Source: CAD feature listing. Evaluate the final solid. Frame: model axes, mm. A direction names the side the tool comes from. Round coordinates to 2 decimals unless told otherwise and drop trailing zeros. Loops run counter-clockwise (first coordinate to the right, second up) from the corner with the lowest first, then second, coordinate; pieces in that order, holes last. Notation, with made-up numbers: (-14, 8.25) -> (25, 8.25) arc R13 ccw to (25, 25.25) -> close; hole circle Ø4 at (46, 35). An arc over 180 degrees is marked (long way). Put each result on its own line as item: value. Start each with the question number.
1. Contact query for flat-ended pins moving along their axis: pin 1 (6 mm diameter, centred on y = 8.5, z = -19.5, fed in from +X); pin 2 (8 mm diameter, centred on y = 22.5, z = 22, fed in from -X); pin 3 (7 mm diameter, centred on x = -59, z = 2, fed in from +Y); pin 4 (3 mm diameter, centred on x = -58.17, z = 35.25, fed in from +Y). Output: stop coordinate, or through.
2. Set-up query: faces 1 (the flat face through (-56.101, 1.689, 47.074)), 2 (the flat face through (-64, 3, -1)). Return all of +Z, -Z, +X, -X, +Y, -Y with unobstructed straight access to the full face (end or side cutting, diameter ignored); none if empty.
3. Cut plane A-A (z = 0). Return the cut outline in (x, y), then the cut area to 3 significant figures.
4. Cut plane B-B (y = 31.5). Return the cut outline in (x, z).
5. Draft query along X for faces 3 (the conical face through (-85.33, 17.02, 0.83)), 4 (the cylindrical face through (-61.913, 1.479, 0.54)), 5 (the cylindrical face through (-59.74, 1.48, 35.9)), 6 (the cylindrical face through (-88.35, 35.92, -0.07)). Return one class per face: pulls with the +X half, pulls with the -X half, needs draft (parallel to the pull), parting line crosses it, or undercut.
6. Material intervals for L1, parallel to Y at x = -65.5, z = -9.5; L2, parallel to Z at x = -70, y = 5; L3, parallel to Y at x = -73.5, z = -21, sorted ascending.
```python
from build123d import *

# Parameters (mm, degrees)
R_VOLUTION1_ANGLE                         = 80
BOSS_EXTRU_1_REACH                        = 122.843
ESQUISSE3_R                               = 4
TROU_POUR_TARAUDAGE_POUR_TROU_TARAUD_M4_D = 3.3
D_GAGEMENT_M31_D                          = 3.4
ESQUISSE8_R                               = 41.654908191
ENL_V_MAT_EXTRU_1_DEPTH                   = 121.842511717
CONG_1_R                                  = 5


with BuildPart() as part:
    # Esquisse1 → Révolution1 (revolve, symmetric)
    with BuildSketch(Plane.XY) as r_volution1_sk:
        Polygon((-61.915329373, 0), (-79, 0), (-95, 43), (-91.799050303, 43), (-76.915329373, 3), (-61.915329373, 3), align=None)
    revolve(axis=Axis((0, 0, 0), (0, 1, 0)), revolution_arc=R_VOLUTION1_ANGLE / 2)
    revolve(r_volution1_sk.sketch, axis=Axis((0, 0, 0), (0, -1, 0)), revolution_arc=R_VOLUTION1_ANGLE / 2)

    # Esquisse3 → Boss.-Extru.1 (add, up to next)
    with BuildSketch(Plane(origin=(0, 43, 0), x_dir=(1, 0, 0), z_dir=(0, 1, 0)), mode=Mode.PRIVATE) as boss_extru_1_sk1:
        with Locations((-90, 0)):
            Circle(ESQUISSE3_R)
    boss_extru_1_tool1 = extrude(boss_extru_1_sk1.sketch, amount=-BOSS_EXTRU_1_REACH, mode=Mode.PRIVATE) - part.part
    add(boss_extru_1_tool1.solids().sort_by_distance((-90, 43, 0))[0])

    # Trou pour taraudage pour trou taraudé M41 (through all)
    with Locations(Plane(origin=(0, 43, 0), x_dir=(1, 0, 0), z_dir=(0, 1, 0))):
        with Locations((-90, 0)):
            Hole(TROU_POUR_TARAUDAGE_POUR_TROU_TARAUD_M4_D / 2)

    # Dégagement M31 (through all)
    with Locations(Plane(origin=(0, 3, 0), x_dir=(1, 0, 0), z_dir=(0, 1, 0))):
        with Locations((-58.168039621, 35.25), (-58.168039621, -35.25)):
            Hole(D_GAGEMENT_M31_D / 2)

    # Esquisse8 → Enlèv. mat.-Extru.1 (cut, through all)
    with BuildSketch(Plane(origin=(0, 0, 0), x_dir=(0, 0, -1), z_dir=(1, 0, 0))):
        with Locations((-61.06482292, 43)):
            Circle(ESQUISSE8_R)
        with Locations((61.06482292, 43)):
            Circle(ESQUISSE8_R)
    extrude(amount=-ENL_V_MAT_EXTRU_1_DEPTH, mode=Mode.SUBTRACT)

    # Congé1
    cong_1_edges = [part.edges().sort_by_distance(p)[0] for p in [
        (-76.915329373, 3, 0),
        (-91.359787942, 43, -19.409914729),
        (-91.359787942, 43, 19.409914729),
        (-47.42989401, 1.5, -39.798406571),
        (-47.42989401, 1.5, 39.798406571),
    ]]
    fillet(cong_1_edges, radius=CONG_1_R)


solid = part.part
```
Solution:
1. pin 1: stops at x = -75.1
1. pin 2: stops at x = -86.38
1. pin 3: stops at y = 3
1. pin 4: passes through
2. face 1: +Z, +X, +Y, -Y
2. face 2: +X, +Y
3. outline: (-95, 43) -> (-91.65, 34) -> (-91.65, 43) -> close; (-88.35, 25.13) -> (-79, 0) -> (-61.92, 0) -> (-61.92, 3) -> (-73.44, 3) arc R5 cw to (-78.13, 6.26) -> (-86, 27.42) -> (-86, 43) -> (-88.35, 43) -> close
3. area: 184 mm^2
4. outline: (-90.71, -1.49) arc R90.72 ccw to (-88.25, -21.03) -> (-84.96, -21.03) arc R87.52 cw to (-87.47, -3.09) arc R4 ccw to (-87.47, 3.09) arc R87.52 cw to (-84.96, 21.03) -> (-88.25, 21.03) arc R90.72 ccw to (-90.71, 1.49) arc R1.65 cw (long way) to start
5. face 3: pulls with the -X half
5. face 4: pulls with the +X half
5. face 5: undercut
5. face 6: undercut
6. L1: y = 0 to 3
6. L2: z = -40.48 to -33.12, 33.12 to 40.48
6. L3: y = 0 to 4
